Geometry: final body of the model. Coordinates: model frame, mm. Face numbers are marked on the shaded views. A direction names the side the tool comes from. Coordinates: 2 decimals unless noted, no trailing zeros. Loops run counter-clockwise (first coordinate to the right, second up) from the corner with the lowest first, then second, coordinate; pieces in that order, holes last. Notation, with made-up numbers: (-30, 1) -> (-24, 1) arc R20 ccw to (-24, 31) -> close; hole circle Ø9 at (-39.75, -23.5). An arc over 180 degrees is marked (long way). One line per item, written item: value. Start each with the question number.
Item 1: Section query B-B on x = 0. Return loops of the section in (y, z), then the cut area to 4 significant figures.
Item 2: Section query D-D on z = -2.5. Return loops of the section in (x, y).
Item 3: Set-up query: the marked faces 4, 5, 6, 7 and 8. Return all of +Z, -Z, +X, -X, +Y, -Y with unobstructed straight access to the full face (end or side cutting, diameter ignored); none if empty.
Item 4: Section query C-C on y = 2.75. Return loops of the section in (x, z), then the cut area to 3 significant figures.
Item 5: Mould query, pull axis X, two halves, no side actions, for the marked faces 1, 2 and 3. Classes: +X half, -X half, draft (parallel to the pull), parting line (faces both ways), or undercut.
Item 6: Ray query, probe 1 along Y at (x, z) = (0, 6.75); probe 2 along Z at (x, y) = (0, 10.5). Return the intervals inside material, ascending. Write a range as from..to.
Item 7: Contact query for flat-ended pins moving along their axis: pin 1 Ø1.5 at (x, y) = (-2.5, 2.5) entering from -Z; pin 2 Ø3 at (x, y) = (-4, 10) entering from -Z; pin 3 Ø2.5 at (y, z) = (3.85, 0) entering from -X. Output: stop coordinate, or through.
Item 8: Section query A-A on z = 0. Return loops of the section in (x, y), then the cut area to 4 significant figures.
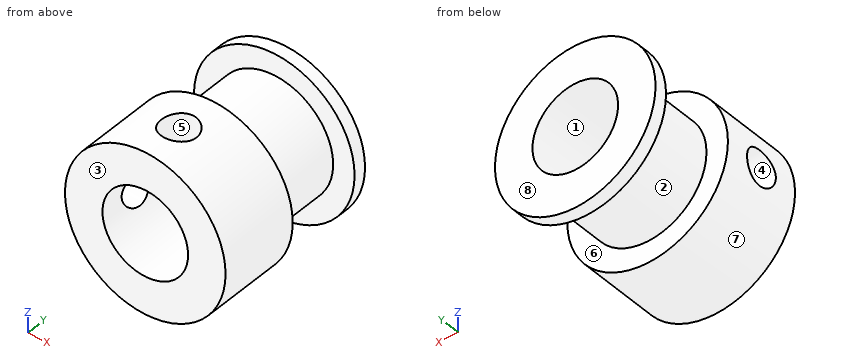
from build123d import *

# Parameters (mm, degrees)
CROQUIS1_R              = 7.5
SALIENTE_EXTRUIR1_DEPTH = 7.7
CROQUIS2_R              = 5.5
SALIENTE_EXTRUIR2_DEPTH = 7.1
CROQUIS3_R              = 7.5
SALIENTE_EXTRUIR3_DEPTH = 1.2
CROQUIS4_R              = 4
CORTAR_EXTRUIR1_DEPTH   = 17
CROQUIS5_W              = 1.65
CROQUIS5_H              = 7.501
MATRIZC1_COUNT          = 2
MATRIZC1_ANGLE          = 90


with BuildPart() as part:
    # Croquis1 → Saliente-Extruir1 (new body)
    with BuildSketch(Plane(origin=(0, 0, 0), x_dir=(1, 0, 0), z_dir=(0, 1, 0))):
        Circle(CROQUIS1_R)
    extrude(amount=SALIENTE_EXTRUIR1_DEPTH)

    # Croquis2 → Saliente-Extruir2 (add)
    with BuildSketch(Plane(origin=(0, 7.7, 0), x_dir=(1, 0, 0), z_dir=(0, 1, 0))):
        Circle(CROQUIS2_R)
    extrude(amount=SALIENTE_EXTRUIR2_DEPTH)

    # Croquis3 → Saliente-Extruir3 (add)
    with BuildSketch(Plane(origin=(0, 14.8, 0), x_dir=(1, 0, 0), z_dir=(0, 1, 0))):
        Circle(CROQUIS3_R)
    extrude(amount=SALIENTE_EXTRUIR3_DEPTH)

    # Croquis4 → Cortar-Extruir1 (cut, through all)
    with BuildSketch(Plane(origin=(0, 16, 0), x_dir=(1, 0, 0), z_dir=(0, 1, 0))):
        Circle(CROQUIS4_R)
    extrude(amount=-CORTAR_EXTRUIR1_DEPTH, mode=Mode.SUBTRACT)

    # Croquis5 → Taladro roscado M31 (definir posicio) (revolve, cut)
    with BuildSketch(Plane(origin=(0, 3.85, 0), x_dir=(0, 1, 0), z_dir=(1, 0, 0))):
        with Locations((0.825, 3.7505)):
            Rectangle(CROQUIS5_W, CROQUIS5_H)
    taladro_roscado_m31_definir_posicio = revolve(axis=Axis((0, 3.85, -6.35), (0, 0, 1)), mode=Mode.SUBTRACT)

    # MatrizC1: Taladro roscado M31 (definir posicio) ×2 about axis
    matrizc1_axis = Axis((0, 7.7, 0), (0, -1, 0))
    for i in range(1, MATRIZC1_COUNT):
        add(taladro_roscado_m31_definir_posicio.rotate(matrizc1_axis, i * MATRIZC1_ANGLE / (MATRIZC1_COUNT - 1)), mode=Mode.SUBTRACT)


solid = part.part
Reply:
1. outline: (0, -7.5) -> (7.7, -7.5) -> (7.7, -5.5) -> (14.8, -5.5) -> (14.8, -7.5) -> (16, -7.5) -> (16, -4) -> (0, -4) -> close; (0, 4) -> (2.2, 4) -> (2.2, 7.5) -> (0, 7.5) -> close; (5.5, 4) -> (16, 4) -> (16, 7.5) -> (14.8, 7.5) -> (14.8, 5.5) -> (7.7, 5.5) -> (7.7, 7.5) -> (5.5, 7.5) -> close
1. area: 72.05 mm²
2. outline: (-7.07, 0) -> (-3.12, 0) -> (-3.12, 16) -> (-7.07, 16) -> (-7.07, 14.8) -> (-4.9, 14.8) -> (-4.9, 7.7) -> (-7.07, 7.7) -> close; (3.12, 0) -> (7.07, 0) -> (7.07, 7.7) -> (4.9, 7.7) -> (4.9, 14.8) -> (7.07, 14.8) -> (7.07, 16) -> (3.12, 16) -> close
3. face 4: -X
3. face 5: +Z
3. face 6: none
3. face 7: +Y, -Y
3. face 8: +Z, -Z, +X, -X, +Y
4. outline: (-7.4, -1.23) arc R7.5 ccw (long way) to (1.23, 7.4) -> (1.23, 3.81) arc R4 cw (long way) to (-3.81, -1.23) -> close; (-7.4, 1.23) -> (-3.81, 1.23) arc R4 cw to (-1.23, 3.81) -> (-1.23, 7.4) arc R7.5 ccw to start
4. area: 109 mm²
5. face 1: undercut
5. face 2: parting line
5. face 3: draft
6. probe 1: y = 0..2.2, 5.5..7.7, 14.8..16
6. probe 2: z = -5.5..-4, 4..5.5
7. pin 1: stops at z = -7.29
7. pin 2: stops at z = -4.9
7. pin 3: stops at x = 3.8
8. outline: (-7.5, 0) -> (-4, 0) -> (-4, 2.2) -> (-7.5, 2.2) -> close; (-7.5, 5.5) -> (-4, 5.5) -> (-4, 16) -> (-7.5, 16) -> (-7.5, 14.8) -> (-5.5, 14.8) -> (-5.5, 7.7) -> (-7.5, 7.7) -> close; (4, 0) -> (7.5, 0) -> (7.5, 7.7) -> (5.5, 7.7) -> (5.5, 14.8) -> (7.5, 14.8) -> (7.5, 16) -> (4, 16) -> close
8. area: 72.05 mm²
